CAD build for the part. Positions are in the model's coordinates, mm. A direction names the side the tool comes from. Give positions to 0.01 mm unless a question says otherwise; leave off trailing zeros. Write each loop counter-clockwise with the first axis right and the second up, starting at its lowest first coordinate (ties: lowest second). Pieces come first, ordered by that corner, then holes. Notation, with made-up numbers: (3.5, 40.25) - (29.5, 40.25) arc R28 ccw to (29.5, 75.25) - close; hole circle Ø3 at (11, 74). An arc over 180 degrees is marked (long way). Answer as a JSON object with one key per item and string values.
from build123d import *

# Parameters (mm, degrees)
SKETCH1_W           = 90
SKETCH1_H           = 400
BOSS_EXTRUDE1_DEPTH = 110
SHELL1_T            = 2
CUT_EXTRUDE2_REACH  = 247.357
SKETCH2_W           = 170
SKETCH2_H           = 340
CUT_EXTRUDE3_REACH  = 302.707
SKETCH5_R           = 20
SKETCH5_R_2         = 2.5
SKETCH6_W           = 70
SKETCH6_H           = 400
BOSS_EXTRUDE2_DEPTH = 2


with BuildPart() as part:
    # Sketch1 → Boss-Extrude1 (new, symmetric)
    with BuildSketch(Plane.XY):
        Rectangle(SKETCH1_W, SKETCH1_H)
    extrude(amount=BOSS_EXTRUDE1_DEPTH, both=True)

    # Shell1 (no face opened: a closed hollow body)
    add(offset(amount=-SHELL1_T, mode=Mode.PRIVATE), mode=Mode.SUBTRACT)

    # Sketch2 → Cut-Extrude2 (cut, up to next)
    with BuildSketch(Plane(origin=(45, 0, 0), x_dir=(0, 0, -1), z_dir=(1, 0, 0)), mode=Mode.PRIVATE) as cut_extrude2_sk1:
        Rectangle(SKETCH2_W, SKETCH2_H)
    cut_extrude2_tool1 = extrude(cut_extrude2_sk1.sketch, amount=-CUT_EXTRUDE2_REACH, mode=Mode.PRIVATE) & part.part
    add(cut_extrude2_tool1.solids().sort_by_distance((45, 0, 0))[0], mode=Mode.SUBTRACT)

    # Sketch5 → Cut-Extrude3 (cut, up to next)
    with BuildSketch(Plane.XY.offset(110), mode=Mode.PRIVATE) as cut_extrude3_sk1:
        with Locations((0, -115)):
            Circle(SKETCH5_R)
    cut_extrude3_tool1 = extrude(cut_extrude3_sk1.sketch, amount=-CUT_EXTRUDE3_REACH, mode=Mode.PRIVATE) & part.part
    # Sketch5 → Cut-Extrude3 (cut, up to next)
    with BuildSketch(Plane.XY.offset(110), mode=Mode.PRIVATE) as cut_extrude3_sk2:
        with Locations((-22.275, -92.725)):
            Circle(SKETCH5_R_2)
    cut_extrude3_tool2 = extrude(cut_extrude3_sk2.sketch, amount=-CUT_EXTRUDE3_REACH, mode=Mode.PRIVATE) & part.part
    # Sketch5 → Cut-Extrude3 (cut, up to next)
    with BuildSketch(Plane.XY.offset(110), mode=Mode.PRIVATE) as cut_extrude3_sk3:
        with Locations((22.275, -92.725)):
            Circle(SKETCH5_R_2)
    cut_extrude3_tool3 = extrude(cut_extrude3_sk3.sketch, amount=-CUT_EXTRUDE3_REACH, mode=Mode.PRIVATE) & part.part
    # Sketch5 → Cut-Extrude3 (cut, up to next)
    with BuildSketch(Plane.XY.offset(110), mode=Mode.PRIVATE) as cut_extrude3_sk4:
        with Locations((-22.275, -137.275)):
            Circle(SKETCH5_R_2)
    cut_extrude3_tool4 = extrude(cut_extrude3_sk4.sketch, amount=-CUT_EXTRUDE3_REACH, mode=Mode.PRIVATE) & part.part
    # Sketch5 → Cut-Extrude3 (cut, up to next)
    with BuildSketch(Plane.XY.offset(110), mode=Mode.PRIVATE) as cut_extrude3_sk5:
        with Locations((22.275, -137.275)):
            Circle(SKETCH5_R_2)
    cut_extrude3_tool5 = extrude(cut_extrude3_sk5.sketch, amount=-CUT_EXTRUDE3_REACH, mode=Mode.PRIVATE) & part.part
    add(cut_extrude3_tool1.solids().sort_by_distance((0, -115, 110))[0], mode=Mode.SUBTRACT)
    add(cut_extrude3_tool2.solids().sort_by_distance((-22.275, -92.725, 110))[0], mode=Mode.SUBTRACT)
    add(cut_extrude3_tool3.solids().sort_by_distance((22.275, -92.725, 110))[0], mode=Mode.SUBTRACT)
    add(cut_extrude3_tool4.solids().sort_by_distance((-22.275, -137.275, 110))[0], mode=Mode.SUBTRACT)
    add(cut_extrude3_tool5.solids().sort_by_distance((22.275, -137.275, 110))[0], mode=Mode.SUBTRACT)

    # Sketch6 → Boss-Extrude2 (add)
    with BuildSketch(Plane(origin=(0, 0, -110), x_dir=(-1, 0, 0), z_dir=(0, 0, -1))):
        with Locations((80, 0)):
            Rectangle(SKETCH6_W, SKETCH6_H)
    extrude(amount=-BOSS_EXTRUDE2_DEPTH)


solid = part.part
(1) 3-axis set-ups, long thin cutter, end or side, ignore diameter. For faces 1 (the face through (2, 200, -2)), 2 (the face through (-1, 3, -108)), 3 (the face through (-45, -3, 3)), 4 (the face through (-1, 3, 110)), 5 (the face through (-4.336, -134.524, 109.014)): which of +Z, -Z, +X, -X, +Y, -Y reach the whole face in a straight line?
Answer key:
{"face 1": "+Z, -Z, +X, -X, +Y", "face 2": "none", "face 3": "+Z, -X, +Y, -Y", "face 4": "+Z, +X, -X, +Y, -Y", "face 5": "+Z"}
(2) Probe L1, parallel to Y at x = 17.5, z = 58.5; L2, parallel to Z at x = -38, y = -112.5; L3, parallel to X at y = 176.5, z = -88. List the from-to ranges inside material, lowest first. Write a range as [from, to].
Answer key:
{"L1": "y = [-200, -198], [198, 200]", "L2": "z = [-110, -108], [108, 110]", "L3": "x = [-45, -43], [43, 45]"}
(3) Saw through at B-B, the plane z = 89. Give the cut face in (x, y), and give its area (3 significant figures).
Answer key:
{"outline": "(-45, -200) - (45, -200) - (45, 200) - (-45, 200) - close; hole (-43, -198) - (43, -198) - (43, 198) - (-43, 198) - close", "area": "1,940 mm²"}
(4) Saw through at D-D, the plane z = -44. Give the cut face in (x, y).
Answer key:
{"outline": "(-45, -200) - (45, -200) - (45, -170) - (43, -170) - (43, -198) - (-43, -198) - (-43, 198) - (43, 198) - (43, 170) - (45, 170) - (45, 200) - (-45, 200) - close"}
(5) Saw through at C-C, the plane y = -161.5. Give the cut face in (x, z).
Answer key:
{"outline": "(-115, -110) - (45, -110) - (45, -85) - (43, -85) - (43, -108) - (-43, -108) - (-43, 108) - (43, 108) - (43, 85) - (45, 85) - (45, 110) - (-45, 110) - (-45, -108) - (-115, -108) - close"}
(6) Saw through at A-A, the plane y = -115. Give the cut face in (x, z), and give its area (3 significant figures).
Answer key:
{"outline": "(-115, -110) - (45, -110) - (45, -85) - (43, -85) - (43, -108) - (-43, -108) - (-43, 108) - (-20, 108) - (-20, 110) - (-45, 110) - (-45, -108) - (-115, -108) - close; (20, 108) - (43, 108) - (43, 85) - (45, 85) - (45, 110) - (20, 110) - close", "area": "944 mm²"}
(7) Pull direction X, two halves, no side cores. Call faces 6 (the face through (45, -3, -96)), 7 (the face through (-1, -198, 2)), 8 (the face through (-80, 3, -108)): pulls with the +X half, pulls with the -X half, needs draft (parallel to the pull), parting line crosses it, or undercut.
Answer key:
{"face 6": "pulls with the +X half", "face 7": "undercut", "face 8": "needs draft"}
(8) Flat gauge pins, fed straight in: P1, Ø12, axis at x = -59, y = -106.5, coming from the +Z side; P2, Ø2, axis at y = -55, z = -35, coming from the -X side; P3, Ø10, axis at y = -17, z = 29, coming from the +X side. Where does each tip first touch, or does it go through?
Answer key:
{"P1": "stops at z = -108", "P2": "stops at x = -45", "P3": "stops at x = -43"}
